Build history of the part. All positions in model axes, mm. Face numbers are marked on the shaded views. A direction names the side the tool comes from. Round coordinates to 2 decimals unless told otherwise and drop trailing zeros. Write each loop counter-clockwise with the first axis right and the second up, starting at its lowest first coordinate (ties: lowest second). Pieces come first, ordered by that corner, then holes. Notation, with made-up numbers: M 86.25,66 L 102.25,66 A23 cw 102.25,103 Z; hole C -15.5,56 d5. An arc over 180 degrees is marked long. Use a Markdown table: item, result.
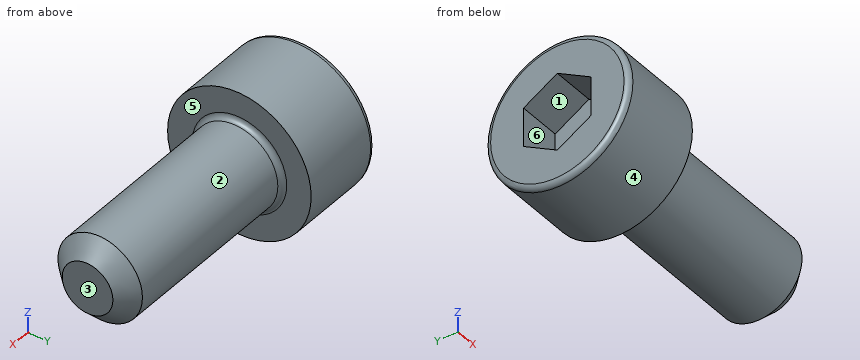
from build123d import *

# Parameters (mm, degrees)
CUT_EXTRUDE_1_DEPTH = 2.5
FILLET_1_R          = 0.3
CHAMFER_1_SIZE      = 1


with BuildPart() as part:
    # Эскиз1 → Повернуть1 (revolve)
    with BuildSketch(Plane.XY):
        Polygon((0, 0), (0, 4.25), (5, 4.25), (5, 2.5), (17, 2.5), (17, 0), align=None)
    revolve(axis=Axis((17, 0, 0), (-1, 0, 0)))

    # Эскиз2 → Вырез-Вытянуть1 (cut)
    with BuildSketch(Plane.ZY):
        Polygon((-1.154700538, 2), (-2.309401077, 0), (-1.154700538, -2), (1.154700538, -2), (2.309401077, 0), (1.154700538, 2), align=None)
    extrude(amount=-CUT_EXTRUDE_1_DEPTH, mode=Mode.SUBTRACT)

    # Скругление1
    fillet_1_edges = [part.edges().sort_by_distance(p)[0] for p in [
        (5, -2.5, 0),
        (0, -4.25, 0),
    ]]
    fillet(fillet_1_edges, radius=FILLET_1_R)

    # Фаска1
    chamfer_1_edges = [part.edges().sort_by_distance(p)[0] for p in [
        (17, -2.5, 0),
    ]]
    chamfer(chamfer_1_edges, length=CHAMFER_1_SIZE)


solid = part.part
Q1. Cut at B-B on x = 12.75. Give the cut face in (y, z).
Response values:
| item | result |
|---|---|
| outline | C 0,0 d5 |
Q2. Drop flat-ended pins along their axis: P1, Ø1.5, axis at x = 4, z = 1, coming from the +Y side; P2, Ø1.5, axis at x = 5, y = -2, coming from the -Z side; P3, Ø5, axis at x = 11, y = 1.5, coming from the +Z side. Give the stop position or say it passes through.
Response values:
| item | result |
|---|---|
| P1 | stops at y = 4.24 |
| P2 | stops at z = -4.06 |
| P3 | stops at z = 2.5 |
Q3. Two-plate mould, pull along Y, no slides. Class the marked faces 1, 2 and 3: +Y half, -Y half, draft (parallel to the pull), parting line (faces both ways), or undercut.
Response values:
| item | result |
|---|---|
| face 1 | undercut |
| face 2 | parting line |
| face 3 | draft |
Q4. Drill centre lines: L1, parallel to X at y = 2.5, z = 2.25; L2, parallel to Y at x = 6, z = 0; L3, parallel to X at y = 0.5, z = -0.75. Where is each one in solid material? Low to high.
Response values:
| item | result |
|---|---|
| L1 | x = 0 to 5 |
| L2 | y = -2.5 to 2.5 |
| L3 | x = 2.5 to 17 |
Q5. Cut at A-A on x = 1.75. Give the cut face in (y, z).
Response values:
| item | result |
|---|---|
| outline | C 0,0 d8.5; hole M -2,-1.15 L 0,-2.31 L 2,-1.15 L 2,1.15 L 0,2.31 L -2,1.15 Z |
Q6. Which spindle directions (+Z, -Z, +X, -X, +Y, -Y) get a long thin tool onto all of the face, cutting with end or side? Do the marked faces 4, 5 and 6. Say none if no direction does.
Response values:
| item | result |
|---|---|
| face 4 | +X, -X |
| face 5 | +X |
| face 6 | -X |
